Part model, mm, in its own coordinate system. A direction names the side the tool comes from. Round coordinates to 2 decimals unless told otherwise and drop trailing zeros. Write each loop counter-clockwise with the first axis right and the second up, starting at its lowest first coordinate (ties: lowest second). Pieces come first, ordered by that corner, then holes. Notation, with made-up numbers: (5, 43) -> (44, 43) arc R19 ccw to (44, 63) -> close; hole circle Ø9 at (15.5, 7.25). An arc over 180 degrees is marked (long way). Use CSV: the item, a comma, the result in double quotes. Start each with the question number.
(1) Saw through at A-A (z = -1). Give the cut face in (x, y) (3 decimals), plus the area to 3 significant figures.
(2) Saw through at C-C (y = -16.5). Give the cut face in (x, z), plus the area to 3 significant figures.
(3) Which spindle directions (+Z, -Z, +X, -X, +Y, -Y) get a long thin tool onto all of the face, cutting with end or side? Do faces 1 (the flat face through (41, -19.685, 0)), 2 (the flat face through (51, -0.635, 0)), 3 (the flat face through (0, -5, 0)). Say none if no direction does.
(4) Probe line 1 (Y direction, x = 67.5, z = -1.7) (3 decimals); line 2 (Y direction, x = -8, z = 2.25) (3 decimals); line 3 (X direction, y = -14, z = 0.6). List the from-to ranges inside material, lowest first. Write a range as [from, to].
(5) Saw through at B-B (x = 56.5). Give the cut face in (y, z) (3 decimals), plus the area to 3 significant figures.
(6) Drop flat-ended pins along their axis: pin 1 (1 mm diameter, centred on y = -6, z = -0.5, fed in from +X); pin 2 (1.5 mm diameter, centred on y = -8, z = 0.5, fed in from -X); pin 3 (2.5 mm diameter, centred on x = -26.5, z = 0, fed in from -Y). Give the stop position or say it passes through.
```python
from build123d import *

# Parameters (mm, degrees)
F1_DEPTH = 2.54


with BuildPart() as f1:
    # F0 (on Top) → F1 (new body, symmetric)
    with BuildSketch(Plane.XY):
        with BuildLine():
            ThreePointArc((-63.5, 8.89), (-60.896179, 2.603821), (-54.61, 0))
            Line((-54.61, 0), (0, 0))
            Line((0, 0), (0, -10.795))
            ThreePointArc((0, -10.795), (2.603821, -17.081179), (8.89, -19.685))
            Line((8.89, -19.685), (73.66, -19.685))
            ThreePointArc((73.66, -19.685), (79.946179, -17.081179), (82.55, -10.795))
            Line((82.55, -10.795), (82.55, -9.525))
            ThreePointArc((82.55, -9.525), (79.946179, -3.238821), (73.66, -0.635))
            Line((73.66, -0.635), (27.942636, -0.635))
            ThreePointArc((27.942636, -0.635), (20.658215, 1.661769), (16.008539, 7.721344))
            Line((16.008539, 7.721344), (15.157828, 10.058656))
            ThreePointArc((15.157828, 10.058656), (10.508152, 16.118231), (3.223731, 18.415))
            Line((3.223731, 18.415), (-54.61, 18.415))
            ThreePointArc((-54.61, 18.415), (-60.896179, 15.811179), (-63.5, 9.525))
            Line((-63.5, 9.525), (-63.5, 8.89))
        make_face()
    extrude(amount=F1_DEPTH, both=True)


solid = f1.part
```
Answers:
1,outline,"(-63.5, 8.89) arc R8.89 ccw to (-54.61, 0) -> (0, 0) -> (0, -10.795) arc R8.89 ccw to (8.89, -19.685) -> (73.66, -19.685) arc R8.89 ccw to (82.55, -10.795) -> (82.55, -9.525) arc R8.89 ccw to (73.66, -0.635) -> (27.943, -0.635) arc R12.7 cw to (16.009, 7.721) -> (15.158, 10.059) arc R12.7 ccw to (3.224, 18.415) -> (-54.61, 18.415) arc R8.89 ccw to (-63.5, 9.525) -> close"
1,area,"2,950 mm²"
2,outline,"(2.07, -2.54) -> (80.48, -2.54) -> (80.48, 2.54) -> (2.07, 2.54) -> close"
2,area,"398 mm²"
3,face 1,"+Z, -Z, +X, -X, -Y"
3,face 2,"+Z, -Z, +X, +Y"
3,face 3,"+Z, -Z, -X, -Y"
4,line 1,"y = [-19.685, -0.635]"
4,line 2,"y = [0, 18.415]"
4,line 3,"x = [0.6, 81.95]"
5,outline,"(-19.685, -2.54) -> (-0.635, -2.54) -> (-0.635, 2.54) -> (-19.685, 2.54) -> close"
5,area,"96.8 mm²"
6,pin 1,"stops at x = 82.02"
6,pin 2,"stops at x = 0"
6,pin 3,"stops at y = 0"
